from build123d import *

# Parameters (mm, degrees)
BOSS_EXTRUDE1_START                                 = -50
BOSS_EXTRUDE1_DEPTH                                 = 4
CSK_FOR_M3_COUNTERSUNK_FLAT_HEAD_SCREW1_D           = 3.2
CSK_FOR_M3_COUNTERSUNK_FLAT_HEAD_SCREW1_CSINK_D     = 6.3
CSK_FOR_M3_COUNTERSUNK_FLAT_HEAD_SCREW1_CSINK_ANGLE = 90
M3_CLEARANCE_HOLE1_D                                = 3.2
FILLET1_R                                           = 5


with BuildPart() as part:
    # Sketch2 → Boss-Extrude1 (new body)
    with BuildSketch(Plane(origin=(0, 0, 0), x_dir=(0, 0, -1), z_dir=(1, 0, 0)).offset(BOSS_EXTRUDE1_START)):
        with BuildLine():
            Line((5, 8), (5, 22.167543842))
            Line((5, 22.167543842), (22.8, 22.167543842))
            ThreePointArc((22.8, 22.167543842), (23.161099135, 21.78998593), (23.515946886, 21.40654671))
            ThreePointArc((23.515946886, 21.40654671), (26.429411238, 19.642162968), (29.833839376, 19.747962631))
            ThreePointArc((29.833839376, 19.747962631), (35.912951138, 17.155172414), (34.109592252, 10.797023497))
            ThreePointArc((34.109592252, 10.797023497), (31.887887506, 8.215289092), (31.429483161, 4.840205393))
            ThreePointArc((31.429483161, 4.840205393), (31.8, 0), (31.429483161, -4.840205393))
            ThreePointArc((31.429483161, -4.840205393), (31.887887506, -8.215289092), (34.109592252, -10.797023497))
            ThreePointArc((34.109592252, -10.797023497), (35.912951138, -17.155172414), (29.833839376, -19.747962631))
            ThreePointArc((29.833839376, -19.747962631), (26.429411238, -19.642162968), (23.515946886, -21.40654671))
            ThreePointArc((23.515946886, -21.40654671), (23.161099135, -21.78998593), (22.8, -22.167543842))
            Line((22.8, -22.167543842), (-22.8, -22.167543842))
            ThreePointArc((-22.8, -22.167543842), (-23.161099135, -21.78998593), (-23.515946886, -21.40654671))
            ThreePointArc((-23.515946886, -21.40654671), (-26.429411238, -19.642162968), (-29.833839376, -19.747962631))
            ThreePointArc((-29.833839376, -19.747962631), (-35.912951138, -17.155172414), (-34.109592252, -10.797023497))
            ThreePointArc((-34.109592252, -10.797023497), (-31.887887506, -8.215289092), (-31.429483161, -4.840205393))
            ThreePointArc((-31.429483161, -4.840205393), (-31.8, 0), (-31.429483161, 4.840205393))
            ThreePointArc((-31.429483161, 4.840205393), (-31.887887506, 8.215289092), (-34.109592252, 10.797023497))
            ThreePointArc((-34.109592252, 10.797023497), (-35.912951138, 17.155172414), (-29.833839376, 19.747962631))
            ThreePointArc((-29.833839376, 19.747962631), (-26.429411238, 19.642162968), (-23.515946886, 21.40654671))
            ThreePointArc((-23.515946886, 21.40654671), (-23.161099135, 21.78998593), (-22.8, 22.167543842))
            Line((-22.8, 22.167543842), (-5, 22.167543842))
            Line((-5, 22.167543842), (-5, 8))
            Line((-5, 8), (5, 8))
        make_face()
    extrude(amount=BOSS_EXTRUDE1_DEPTH)

    # CSK for M3 Countersunk Flat Head Screw1 (through all)
    with Locations(Plane.ZY.offset(50)):
        with Locations((-31.40127386, 15), (-31.40127386, -15), (31.40127386, 15), (31.40127386, -15)):
            CounterSinkHole(CSK_FOR_M3_COUNTERSUNK_FLAT_HEAD_SCREW1_D / 2, CSK_FOR_M3_COUNTERSUNK_FLAT_HEAD_SCREW1_CSINK_D / 2, counter_sink_angle=CSK_FOR_M3_COUNTERSUNK_FLAT_HEAD_SCREW1_CSINK_ANGLE)

    # M3 Clearance Hole1 (through all)
    with Locations(Plane.ZY.offset(50)):
        with Locations((-8.838834765, 8.838834765), (-8.838834765, -8.838834765), (8.838834765, -8.838834765), (8.838834765, 8.838834765)):
            Hole(M3_CLEARANCE_HOLE1_D / 2)

    # Fillet1
    fillet1_edges = [part.edges().sort_by_distance(p)[0] for p in [
        (-48, 8, 5),
        (-48, 8, -5),
    ]]
    fillet(fillet1_edges, radius=FILLET1_R - 0.0001)  # a hair under: the kernel refuses the full size


solid = part.part
Part model, mm, in its own coordinate system. A direction names the side the tool comes from. Give positions to 0.01 mm unless a question says otherwise; leave off trailing zeros. Write each loop counter-clockwise with the first axis right and the second up, starting at its lowest first coordinate (ties: lowest second). Pieces come first, ordered by that corner, then holes.
1) Cut at C-C on x = -47.8. State how many separate pieces and enclosed holes the cut face has, then the cut area to 3 significant figures.
Resolved:
separate pieces: 1
enclosed holes: 8
area: 2,690 mm2
2) Cut at D-D on y = 0. Write the cut outline in (x, z), then the cut area to 3 significant figures.
Resolved:
outline: (-50, -31.8) - (-46, -31.8) - (-46, 31.8) - (-50, 31.8) - close
area: 254 mm2
3) Two-plate mould, pull along Y, no slides. Class faces 3 (the face through (-48, 22.168, -14)), 4 (the face through (-48.028, 8.171, 31.868)), 5 (the face through (-46, 0, -1)): released by +Y, released by -Y, zero draft, split by the parting line, or undercut.
Resolved:
face 3: released by +Y
face 4: undercut
face 5: zero draft
4) Pin check, flat tips, straight feed: pin 1 (1.2 mm diameter, centred on x = -47.5, y = 19, fed in from +Z); pin 2 (3.5 mm diameter, centred on y = -15, z = 31.4, fed in from -X); pin 3 (2.5 mm diameter, centred on y = -15, z = -31.4, fed in from +X); pin 4 (1 mm diameter, centred on x = -47, y = -6.5, fed in from +Z). Stop position of each tip, or through.
Resolved:
pin 1: stops at z = 35.07
pin 2: stops at x = -48.6
pin 3: passes through
pin 4: stops at z = 31.49
5) Cut at A-A on y = 15. Write the cut outline in (x, z), then the cut area to 3 significant figures.
Resolved:
outline: (-50, -36.4) - (-46, -36.4) - (-46, -33) - (-48.45, -33) - (-50, -34.55) - close; (-50, -28.25) - (-48.45, -29.8) - (-46, -29.8) - (-46, -5) - (-50, -5) - close; (-50, 5) - (-46, 5) - (-46, 29.8) - (-48.45, 29.8) - (-50, 28.25) - close; (-50, 34.55) - (-48.45, 33) - (-46, 33) - (-46, 36.4) - (-50, 36.4) - close
area: 221 mm2
6) Cut at B-B on y = -15. Write the cut outline in (x, z).
Resolved:
outline: (-50, -36.4) - (-46, -36.4) - (-46, -33) - (-48.45, -33) - (-50, -34.55) - close; (-50, -28.25) - (-48.45, -29.8) - (-46, -29.8) - (-46, 29.8) - (-48.45, 29.8) - (-50, 28.25) - close; (-50, 34.55) - (-48.45, 33) - (-46, 33) - (-46, 36.4) - (-50, 36.4) - close
7) Which spindle directions (+Z, -Z, +X, -X, +Y, -Y) get a long thin tool onto all of the face, cutting with end or side? Do faces 1 (the face through (-48.03, -19.63, -26.48)), 2 (the face through (-48, 9, 3)). Say none if no direction does.
Resolved:
face 1: +X, -X, -Y
face 2: +X, -X, +Y
8) Probe L1, parallel to Z at x = -46.7, y = -15; L2, parallel to Z at x = -46.85, y = 15; L3, parallel to Z at x = -49.05, y = -7.5. List the from-to ranges inside material, lowest first.
Resolved:
L1: z = -36.4 to -33, -29.8 to 29.8, 33 to 36.4
L2: z = -36.4 to -33, -29.8 to -5, 5 to 29.8, 33 to 36.4
L3: z = -31.62 to -9.71, -7.96 to 7.96, 9.71 to 31.62
